Design review of the part built by this model. Coordinates are the model's own, in mm. Round coordinates to 2 decimals unless told otherwise and drop trailing zeros. Order: outer loops, then holes, each group sorted by start corner. A loop starts at its lowest first (then second) coordinate and runs counter-clockwise, first axis right, second up. Notation, with made-up numbers: (70, 9) - (128, 9) arc R18 ccw to (128, 41) - close; hole circle Ø11 at (36.25, 10). An arc over 180 degrees is marked (long way). Answer as a JSON object with one key per item and string values. Group by question number.
from build123d import *

# Parameters (mm, degrees)
F0_W          = 7.5
F0_H          = 35
F0_H_2        = 25
F1_DEPTH      = 7.5
F1_DEPTH_BACK = 7.5
F2_R          = 7.49999


# Not quite as in the source:
# - a fillet or chamfer is up to 0.001 mm smaller than in the source, because OpenCascade refuses the exact size


with BuildPart() as f1:
    # F0 (on Front) → F1 (new body, two sides)
    with BuildSketch(Plane.XZ) as f1_sk:
        Polygon((7.5, -12.5), (7.5, 12.5), (0, 12.5), (-7.5, 12.5), (-7.5, -12.5), align=None)
        with Locations((3.75, 30)):
            Rectangle(F0_W, F0_H)
        with Locations((-3.75, 60)):
            Rectangle(F0_W, F0_H_2)
        with Locations((3.75, 60)):
            Rectangle(F0_W, F0_H_2)
        with Locations((-3.75, 30)):
            Rectangle(F0_W, F0_H)
    extrude(amount=F1_DEPTH)
    extrude(f1_sk.sketch, amount=-F1_DEPTH_BACK)

    # F2 (radius 7.5 in the source; OpenCascade refuses exactly that, so slightly less here)
    f2_edges = [f1.edges().sort_by_distance(p)[0] for p in [
        (-7.5, -7.5, 30),
        (7.5, -7.5, 30),
        (-7.5, 7.5, 30),
        (7.5, 7.5, 30),
    ]]
    fillet(f2_edges, radius=F2_R)


solid = f1.part
1. To check wall thickness, follow line 1 (X direction, y = -0.5, z = 13); line 2 (Y direction, x = -3.5, z = -1.5); line 3 (X direction, y = -6, z = 51). State the ranges of each line that lie inside material, in increasing order. Write a range as from..to.
2. Take a section at B-B, the plane y = -4.5. Give the boundary of the cut face in (x, z).
3. Take a section at C-C, the plane x = -2. Give the boundary of the cut face in (y, z), then the cut area to 3 significant figures.
4. Clearance check with flat-ended pins moving along their axes: P1, Ø1.5, axis at y = 4, z = 53.5, coming from the +X side; P2, Ø2, axis at y = -4.5, z = 22, coming from the +X side; P3, Ø1.5, axis at y = 2.5, z = -0.5, coming from the -X side. State where each tip first meets the part, or that it passes through.
Response values:
{
 "1": {"line 1": "-7.48..7.48", "line 2": "-6.63..6.63", "line 3": "-4.5..4.5"},
 "2": {"outline": "(-6, -12.5) - (6, -12.5) - (6, 72.5) - (-6, 72.5) - close"},
 "3": {"outline": "(-7.23, -12.5) - (7.23, -12.5) - (7.23, 72.5) - (-7.23, 72.5) - close", "area": "1,230 mm2"},
 "4": {"P1": "x = 6.76", "P2": "x = 6.63", "P3": "x = -7.29"}
}
